Can you work these out from the model? Positions are in its coordinate system, mm. Face numbers are marked on the shaded views. A direction names the side the tool comes from. Coordinates: 2 decimals unless noted, no trailing zeros. Loops run counter-clockwise (first coordinate to the right, second up) from the corner with the lowest first, then second, coordinate; pieces in that order, holes last.
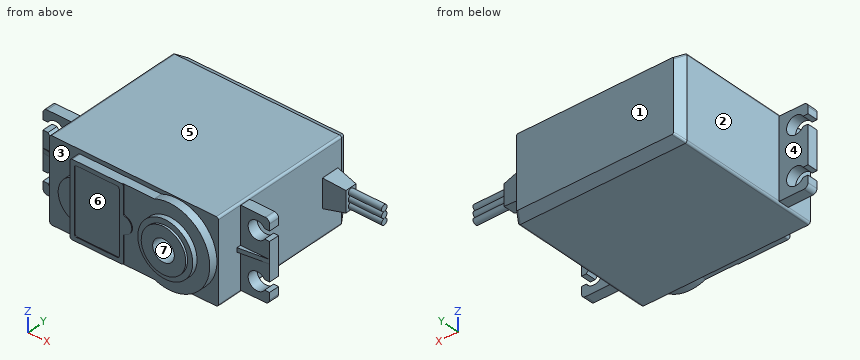
```python
from build123d import *
from OCP.BRepFilletAPI import BRepFilletAPI_MakeChamfer

# Parameters (mm, degrees)
SKETCH_1_W       = 40.5
SKETCH_1_H       = 19.8
BODY_DEPTH       = 36.5
CHAMFER_1_SIZE   = 2.2
CHAMFER_1_SIZE2  = 1.4
FILLET_1_R       = 0.5
MOUNT_DEPTH      = 2.5
EXTRUDE_3_DEPTH  = 0.5
EXTRUDE_4_DEPTH  = 2
SKETCH_5_W       = 10.8
SKETCH_5_H       = 15.84
EXTRUDE_5_DEPTH  = 0.2
SKETCH_6_R       = 6.6
EXTRUDE_6_DEPTH  = 1.2
SKETCH_7_R       = 5.35
EXTRUDE_7_DEPTH  = 0.5
SKETCH_8_R       = 2.6
SHAFT_HOLE_DEPTH = 10
FILLET_2_R       = 0.5
SKETCH_11_R      = 0.75
EXTRUDE_10_DEPTH = 8


with BuildPart() as part:
    # Эскиз1 → Body (new body)
    with BuildSketch(Plane(origin=(0, 0, 0), x_dir=(1, 0, 0), z_dir=(0, 1, 0))):
        Rectangle(SKETCH_1_W, SKETCH_1_H)
    extrude(amount=BODY_DEPTH)

    # Фаска1: one chamfer whose edges measure the first distance from different faces: ONE call of the kernel's chamfer builder (chamfer() names one face for all edges)
    chamfer_1_edges_1 = [part.edges().sort_by_distance(p)[0] for p in [
        (20.25, 36.5, 0),
    ]]
    chamfer_1_side_1 = [part.faces().sort_by_distance(p)[0] for p in [
        (20.25, 18.25, 0),
    ]]
    chamfer_1_edges_2 = [part.edges().sort_by_distance(p)[0] for p in [
        (0, 36.5, -9.9),
    ]]
    chamfer_1_side_2 = [part.faces().sort_by_distance(p)[0] for p in [
        (0, 18.25, -9.9),
    ]]
    chamfer_1_edges_3 = [part.edges().sort_by_distance(p)[0] for p in [
        (-20.25, 36.5, 0),
    ]]
    chamfer_1_side_3 = [part.faces().sort_by_distance(p)[0] for p in [
        (-20.25, 18.25, 0),
    ]]
    chamfer_1_edges_4 = [part.edges().sort_by_distance(p)[0] for p in [
        (0, 36.5, 9.9),
    ]]
    chamfer_1_side_4 = [part.faces().sort_by_distance(p)[0] for p in [
        (0, 18.25, 9.9),
    ]]
    chamfer_1 = BRepFilletAPI_MakeChamfer(part.part.solid().wrapped)
    for e in chamfer_1_edges_1:
        chamfer_1.Add(CHAMFER_1_SIZE, CHAMFER_1_SIZE2, e.wrapped, chamfer_1_side_1[0].wrapped)  # the first distance lies on this face
    for e in chamfer_1_edges_2:
        chamfer_1.Add(CHAMFER_1_SIZE, CHAMFER_1_SIZE2, e.wrapped, chamfer_1_side_2[0].wrapped)  # the first distance lies on this face
    for e in chamfer_1_edges_3:
        chamfer_1.Add(CHAMFER_1_SIZE, CHAMFER_1_SIZE2, e.wrapped, chamfer_1_side_3[0].wrapped)  # the first distance lies on this face
    for e in chamfer_1_edges_4:
        chamfer_1.Add(CHAMFER_1_SIZE, CHAMFER_1_SIZE2, e.wrapped, chamfer_1_side_4[0].wrapped)  # the first distance lies on this face
    add(Compound.cast(chamfer_1.Shape()), mode=Mode.REPLACE)

    # Скругление1
    # the kernel refuses this fillet: 0.5 mm, written as the material it takes off along each edge
    with BuildSketch(Plane(origin=(-20.25, -1.25, 9.9), x_dir=(1, 0, 0), z_dir=(0, 1, 0)), Plane(origin=(-20.25, -1.25, -9.9), x_dir=(0, 0, 1), z_dir=(0, 1, 0))) as fillet_1_piece_1:
        with BuildLine():
            CenterArc((FILLET_1_R, FILLET_1_R), FILLET_1_R, 180, 90)
            Line((0, FILLET_1_R), (0, 0))
            Line((0, 0), (FILLET_1_R, 0))
        make_face()
    extrude(amount=36.8, mode=Mode.SUBTRACT)
    with BuildSketch(Plane(origin=(20.25, -1.25, -9.9), x_dir=(0, 0, 1), z_dir=(0, 1, 0)), Plane(origin=(20.25, -1.25, 9.9), x_dir=(-1, 0, 0), z_dir=(0, 1, 0))) as fillet_1_piece_2:
        with BuildLine():
            CenterArc((FILLET_1_R, -FILLET_1_R), FILLET_1_R, 90, 90)
            Line((0, -FILLET_1_R), (0, 0))
            Line((0, 0), (FILLET_1_R, 0))
        make_face()
    extrude(amount=36.8, mode=Mode.SUBTRACT)
    with BuildSketch(Plane(origin=(20.689497717, 33.609360731, -10.339497717), x_dir=(0.25395078633508533, -0.3990655213836877, 0.8810537485094523), z_dir=(-0.47301616487963943, 0.7433111162394352, 0.47301616487964004)), Plane(origin=(20.689497717, 33.609360731, 10.339497717), x_dir=(-0.8810537485094526, -0.39906552138369156, 0.25395078633507817), z_dir=(-0.47301616487963943, 0.7433111162394352, -0.47301616487964004))) as fillet_1_piece_3:
        with BuildLine():
            CenterArc((FILLET_1_R * 0.743311116239, -FILLET_1_R), FILLET_1_R, 90, 73.247664886)
            Line((-FILLET_1_R * 0.21424849821, -FILLET_1_R * 0.711764705882), (0, 0))
            Line((0, 0), (FILLET_1_R * 0.743311116239, 0))
        make_face()
    extrude(amount=4.818007508, mode=Mode.SUBTRACT)
    with BuildSketch(Plane(origin=(-20.689497717, 33.609360731, -10.339497717), x_dir=(-0.25395078633507856, -0.3990655213836921, 0.8810537485094524), z_dir=(0.47301616487963943, 0.7433111162394352, 0.47301616487964004)), Plane(origin=(-20.689497717, 33.609360731, 10.339497717), x_dir=(0.8810537485094527, -0.3990655213836916, 0.25395078633507817), z_dir=(0.47301616487963943, 0.7433111162394352, -0.47301616487964004))) as fillet_1_piece_4:
        with BuildLine():
            CenterArc((FILLET_1_R * 0.743311116239, FILLET_1_R), FILLET_1_R, 196.752335114, 73.247664886)
            Line((-FILLET_1_R * 0.21424849821, FILLET_1_R * 0.711764705882), (0, 0))
            Line((0, 0), (FILLET_1_R * 0.743311116239, 0))
        make_face()
    extrude(amount=4.818007508, mode=Mode.SUBTRACT)

    # Эскиз2 → Mount (add)
    with BuildSketch(Plane(origin=(0, 6.2, 0), x_dir=(-1, 0, 0), z_dir=(0, -1, 0))):
        with BuildLine():
            Line((-26.2, 9.472835762), (26.2, 9.472835762))
            ThreePointArc((26.2, 9.472835762), (26.907106781, 9.179942543), (27.2, 8.472835762))
            Line((27.2, 8.472835762), (27.2, 6.8))
            Line((27.2, 6.8), (26.016590212, 6.8))
            ThreePointArc((26.016590212, 6.8), (22.05, 5.65), (26.016590212, 4.5))
            Line((26.016590212, 4.5), (27.2, 4.5))
            Line((27.2, 4.5), (27.2, -4.5))
            Line((27.2, -4.5), (26.016590212, -4.5))
            ThreePointArc((26.016590212, -4.5), (22.05, -5.65), (26.016590212, -6.8))
            Line((26.016590212, -6.8), (27.2, -6.8))
            Line((27.2, -6.8), (27.2, -8.4))
            ThreePointArc((27.2, -8.4), (26.907106781, -9.107106781), (26.2, -9.4))
            Line((26.2, -9.4), (-26.2, -9.4))
            ThreePointArc((-26.2, -9.4), (-26.907106781, -9.107106781), (-27.2, -8.4))
            Line((-27.2, -8.4), (-27.2, -6.8))
            Line((-27.2, -6.8), (-26.016590212, -6.8))
            ThreePointArc((-26.016590212, -6.8), (-22.05, -5.65), (-26.016590212, -4.5))
            Line((-26.016590212, -4.5), (-27.2, -4.5))
            Line((-27.2, -4.5), (-27.2, 4.5))
            Line((-27.2, 4.5), (-26.016590212, 4.5))
            ThreePointArc((-26.016590212, 4.5), (-22.05, 5.65), (-26.016590212, 6.8))
            Line((-26.016590212, 6.8), (-27.2, 6.8))
            Line((-27.2, 6.8), (-27.2, 8.472835762))
            ThreePointArc((-27.2, 8.472835762), (-26.907106781, 9.179942543), (-26.2, 9.472835762))
        make_face()
    extrude(amount=-MOUNT_DEPTH)

    # Эскиз3 → Бобышка-Вытянуть3 (add, symmetric)
    with BuildSketch(Plane.XY):
        Polygon((-27.2, 6.2), (-20.25, 6.2), (-20.25, 5.2), align=None)
        Polygon((20.25, 5.2), (27.2, 6.2), (20.25, 6.2), align=None)
    extrude(amount=EXTRUDE_3_DEPTH, both=True)

    # Эскиз4 → Бобышка-Вытянуть4 (add)
    with BuildSketch(Plane.XZ):
        with BuildLine():
            Line((-13.452560024, -8.92), (-13.452560024, -4.6))
            ThreePointArc((-13.452560024, -4.6), (-16.49296823, 0), (-13.452560024, 4.6))
            Line((-13.452560024, 4.6), (-13.452560024, 8.92))
            Line((-13.452560024, 8.92), (6.568139057, 8.92))
            ThreePointArc((6.568139057, 8.92), (19.9, 0), (6.568139057, -8.92))
            Line((6.568139057, -8.92), (-13.452560024, -8.92))
        make_face()
    extrude(amount=EXTRUDE_4_DEPTH)

    # Эскиз5 → Бобышка-Вытянуть5 (add)
    with BuildSketch(Plane.XZ.offset(2)):
        with BuildLine():
            Line((-13.452560024, 8.92), (-0.652560024, 8.92))
            Line((-0.652560024, 8.92), (-0.652560024, 2))
            ThreePointArc((-0.652560024, 2), (1.347439976, 0), (-0.652560024, -2))
            Line((-0.652560024, -2), (-0.652560024, -8.92))
            Line((-0.652560024, -8.92), (-13.452560024, -8.92))
            Line((-13.452560024, -8.92), (-13.452560024, 8.92))
        make_face()
        with Locations((-7.052560024, 0)):
            Rectangle(SKETCH_5_W, SKETCH_5_H, mode=Mode.SUBTRACT)
    extrude(amount=EXTRUDE_5_DEPTH)

    # Эскиз6 → Бобышка-Вытянуть6 (add)
    with BuildSketch(Plane.XZ.offset(2)):
        with Locations(Location((10.25, 0, 0), (0, 0, 270))):
            Circle(SKETCH_6_R)
    extrude(amount=EXTRUDE_6_DEPTH)

    # Эскиз7 → Бобышка-Вытянуть7 (add)
    with BuildSketch(Plane.XZ.offset(3.2)):
        with Locations(Location((10.25, 0, 0), (0, 0, 270))):
            Circle(SKETCH_7_R)
    extrude(amount=EXTRUDE_7_DEPTH)

    # Эскиз8 → Shaft hole (cut)
    with BuildSketch(Plane.XZ.offset(3.7)):
        with Locations(Location((10.25, 0, 0), (0, 0, 270))):
            Circle(SKETCH_8_R)
    extrude(amount=-SHAFT_HOLE_DEPTH, mode=Mode.SUBTRACT)

    # Скругление2
    fillet_2_edges = [part.edges().sort_by_distance(p)[0] for p in [
        (-13.452560024, -1.1, 8.92),
        (-0.652560024, -2.1, 2),
        (-0.652560024, -2.1, -2),
        (-0.652560024, -2.1, 8.92),
        (-0.652560024, -2.1, -8.92),
        (-13.452560024, -1.1, -8.92),
        (-1.652560024, -2.1, 7.92),
        (-1.652560024, -2.1, -7.92),
        (-12.452560024, -2.1, 7.92),
        (-12.452560024, -2.1, -7.92),
    ]]
    fillet(fillet_2_edges, radius=FILLET_2_R)

    # Эскиз10 → Rubber section 0
    with BuildSketch(Plane(origin=(25.25, 0, 0), x_dir=(0, 0, -1), z_dir=(1, 0, 0))):
        with BuildLine():
            Line((-2.5, 29.75), (2.5, 29.75))
            Line((2.5, 29.75), (2.5, 32.55))
            Line((2.5, 32.55), (-2.5, 32.55))
            Line((-2.5, 32.55), (-2.5, 29.75))
        make_face()
    # Эскиз9 → Rubber section 1
    with BuildSketch(Plane(origin=(20.25, 0, 0), x_dir=(0, 0, -1), z_dir=(1, 0, 0))):
        with BuildLine():
            Line((-3.4, 33.3), (3.4, 33.3))
            Line((3.4, 33.3), (3.4, 29))
            Line((3.4, 29), (-3.4, 29))
            Line((-3.4, 29), (-3.4, 33.3))
        make_face()
    loft()

    # Эскиз11 → Бобышка-Вытянуть10 (add)
    with BuildSketch(Plane(origin=(25.25, 0, 0), x_dir=(0, 0, -1), z_dir=(1, 0, 0))):
        with Locations(Location((0, 31.150503064, 0), (0, 0, 180))):
            Circle(SKETCH_11_R)
        with Locations(Location((1.509999917, 31.15000331, 0), (0, 0, 180))):
            Circle(SKETCH_11_R)
        with Locations(Location((-1.509999915, 31.149996646, 0), (0, 0, 180))):
            Circle(SKETCH_11_R)
    extrude(amount=EXTRUDE_10_DEPTH)


solid = part.part
```
(1) Which directions (+Z, -Z, +X, -X, +Y, -Y) give clear straight access to the entire face, cutting with the end or side of a thin tool? Please do the marked faces 1, 2 and 3.
Check values:
face 1: +Z, -Z, +X, -X, +Y
face 2: +Z, -Z, -X, +Y
face 3: -Y
(2) I want a section at C-C on x = 10.25. Write out the boundary of the cut face in (y, z), then the cut area to 3 significant figures.
Check values:
outline: (-3.7, -5.35) - (-3.2, -5.35) - (-3.2, -6.6) - (-2, -6.6) - (-2, -9.65) - (0, -9.65) - (0, -9.9) - (34.3, -9.9) - (36.5, -8.5) - (36.5, 8.5) - (34.3, 9.9) - (0, 9.9) - (0, 9.65) - (-2, 9.65) - (-2, 6.6) - (-3.2, 6.6) - (-3.2, 5.35) - (-3.7, 5.35) - (-3.7, 2.6) - (6.3, 2.6) - (6.3, -2.6) - (-3.7, -2.6) - close
area: 727 mm2
(3) If I drill on probe 1 along Z at (x, y) = (-24.2, 6.8); probe 2 along X at (y, z) = (24, -3.25); probe 3 along Y at (x, z) = (23.5, -8.5), over which ranges is the centre line in solid material (lowest first)?
Check values:
probe 1: z = -9.47 to -7.8, -3.5 to 3.5, 7.8 to 9.4
probe 2: x = -20.25 to 20.25
probe 3: y = 6.2 to 8.7
(4) I want a section at A-A on x = -24.2. Write out the boundary of the cut face in (y, z).
Check values:
outline: (5.77, -0.5) - (6.2, -0.5) - (6.2, -3.5) - (8.7, -3.5) - (8.7, 3.5) - (6.2, 3.5) - (6.2, 0.5) - (5.77, 0.5) - close; (6.2, -9.47) - (8.7, -9.47) - (8.7, -7.8) - (6.2, -7.8) - close; (6.2, 7.8) - (8.7, 7.8) - (8.7, 9.4) - (6.2, 9.4) - close
(5) I want a section at D-D on y = 3. Write out the boundary of the cut face in (x, z), then the cut area to 3 significant figures.
Check values:
outline: (-20.25, -9.4) arc R0.5 ccw to (-19.75, -9.9) - (19.75, -9.9) arc R0.5 ccw to (20.25, -9.4) - (20.25, 9.4) arc R0.5 ccw to (19.75, 9.9) - (-19.75, 9.9) arc R0.5 ccw to (-20.25, 9.4) - close; hole circle Ø5.2 at (10.25, 0)
area: 780 mm2
(6) I'm going to push flat-ended pins straight in: pin 1 (1 mm diameter, centred on y = 13, z = -7.5, fed in from +X); pin 2 (6 mm diameter, centred on x = 9, z = 0.5, fed in from -Y); pin 3 (1.8 mm diameter, centred on y = -1, z = 3, fed in from -X); pin 4 (2.5 mm diameter, centred on x = -4.5, y = -1.5, fed in from -Z). Where does each tip first touch, or does it pass through?
Check values:
pin 1: stops at x = 20.25
pin 2: stops at y = -3.7
pin 3: stops at x = -16.03
pin 4: stops at z = -8.92
(7) If we mould it in two halves opening along Z, with no side actions, what happens to the marked faces 4, 5, 6 and 7? For each: released by +Z, released by -Z, zero draft, split by the parting line, or undercut.
Check values:
face 4: zero draft
face 5: released by +Z
face 6: undercut
face 7: undercut
